Geometry: see drawing. Coordinates: mm, zero at the bounding-box minimum. A direction names the side the tool comes from. Round coordinates to 2 decimals unless told otherwise and drop trailing zeros. Order: outer loops, then holes, each group sorted by start corner. A loop starts at its lowest first (then second) coordinate and runs counter-clockwise, first axis right, second up. Notation, with made-up numbers: (80, -30.5) -> (86, -30.5) arc R20 ccw to (86, 8.5) -> close; hole circle Ø3 at (24, -30.5). An arc over 180 degrees is marked (long way). Use a Markdown table: item, result.
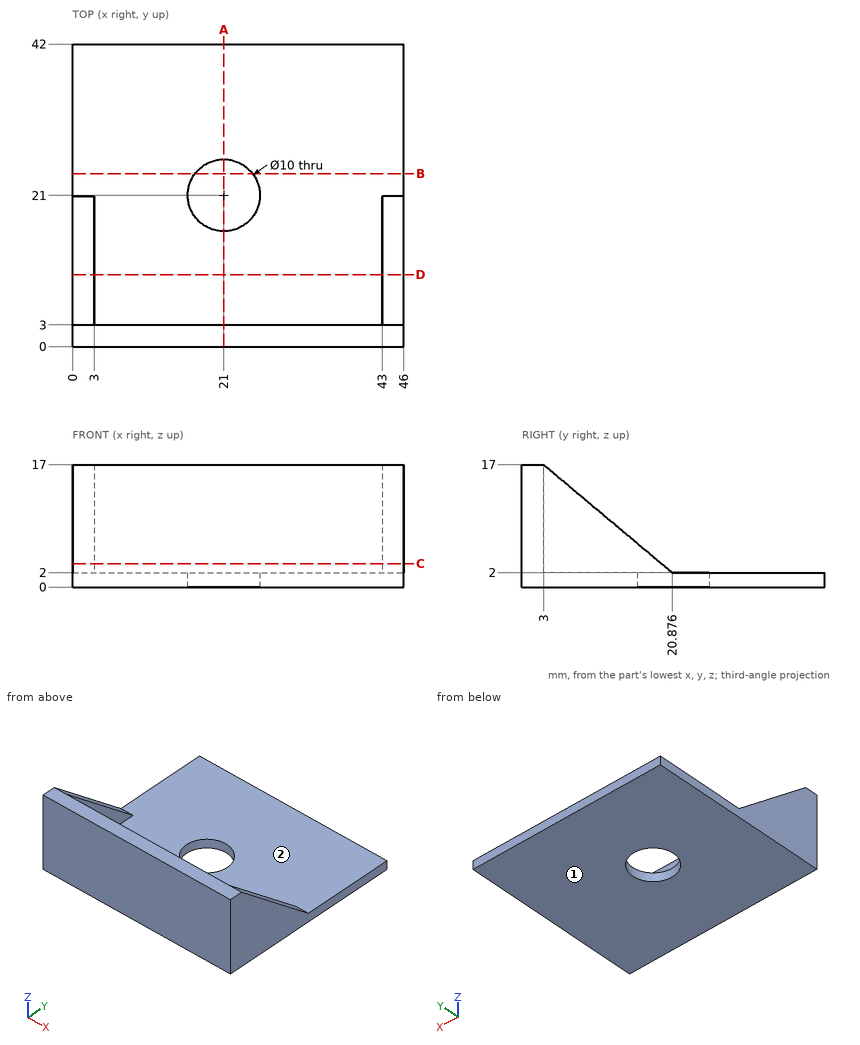
1) Ray query, probe 1 along X at (y, z) = (4.5, 11.25); probe 2 along Y at (x, z) = (21, 1.55); probe 3 along Y at (x, z) = (35.5, 9.75). Return the intervals inside material, ascending.
Answer key:
| item | result |
|---|---|
| probe 1 | x = 0 to 3, 43 to 46 |
| probe 2 | y = 0 to 16, 26 to 42 |
| probe 3 | y = 0 to 3 |
2) Cut plane C-C on z = 3.25. Return loops of the section in (x, y), and give its area (3 significant figures).
Answer key:
| item | result |
|---|---|
| outline | (0, 0) -> (46, 0) -> (46, 19.39) -> (43, 19.39) -> (43, 3) -> (3, 3) -> (3, 19.39) -> (0, 19.39) -> close |
| area | 236 mm^2 |
3) Set-up query: the marked faces 1 and 2. Return all of +Z, -Z, +X, -X, +Y, -Y with unobstructed straight access to the full face (end or side cutting, diameter ignored); none if empty.
Answer key:
| item | result |
|---|---|
| face 1 | -Z, +X, -X, +Y, -Y |
| face 2 | +Z, +Y |
4) Contact query for flat-ended pins moving along their axis: P1, Ø5, axis at x = 36.5, y = 15, coming from the +Z side; P2, Ø4.5, axis at x = 31, z = 8, coming from the +Y side. Output: stop coordinate, or through.
Answer key:
| item | result |
|---|---|
| P1 | stops at z = 2 |
| P2 | stops at y = 3 |
5) Cut plane D-D on y = 10. Return loops of the section in (x, z), and give its area (3 significant figures).
Answer key:
| item | result |
|---|---|
| outline | (0, 0) -> (46, 0) -> (46, 11.13) -> (43, 11.13) -> (43, 2) -> (3, 2) -> (3, 11.13) -> (0, 11.13) -> close |
| area | 147 mm^2 |
6) Cut plane B-B on y = 24. Return loops of the section in (x, z).
Answer key:
| item | result |
|---|---|
| outline | (0, 0) -> (17, 0) -> (17, 2) -> (0, 2) -> close; (25, 0) -> (46, 0) -> (46, 2) -> (25, 2) -> close |
7) Cut plane A-A on x = 21. Return loops of the section in (y, z).
Answer key:
| item | result |
|---|---|
| outline | (0, 0) -> (16, 0) -> (16, 2) -> (3, 2) -> (3, 17) -> (0, 17) -> close; (26, 0) -> (42, 0) -> (42, 2) -> (26, 2) -> close |
